```python
from build123d import *

# Parameters (mm, degrees)
EXTRUDE_THIN1_DEPTH = 317.5
FILLET1_R           = 1.27


with BuildPart() as part:
    # Sketch1 → Extrude-Thin1 (new body)
    with BuildSketch(Plane.XY):
        with BuildLine():
            Line((0, 31.75), (-11.90625, 31.75))
            ThreePointArc((-11.90625, 31.75), (-15.756503047, 28.743813262), (-13.773897059, 24.279411765))
            ThreePointArc((-13.773897059, 24.279411765), (-6.608099772, 17.466390137), (-3.96875, 7.9375))
            Line((-3.96875, 7.9375), (-4.7625, 7.9375))
            ThreePointArc((-4.7625, 7.9375), (-7.540625, 5.159375), (-4.7625, 2.38125))
            Line((-4.7625, 2.38125), (-3.96875, 2.38125))
            Line((-3.96875, 2.38125), (-3.96875, 0))
            Line((-3.96875, 0), (0, 0))
            Line((0, 0), (0, 1.27))
            Line((0, 1.27), (-2.69875, 1.27))
            Line((-2.69875, 1.27), (-2.69875, 3.65125))
            Line((-2.69875, 3.65125), (-4.7625, 3.65125))
            ThreePointArc((-4.7625, 3.65125), (-6.270625, 5.159375), (-4.7625, 6.6675))
            Line((-4.7625, 6.6675), (-2.7395407, 6.6675))
            ThreePointArc((-2.7395407, 6.6675), (-5.200957167, 17.569762939), (-13.17625, 25.4))
            ThreePointArc((-13.17625, 25.4), (-14.524422072, 28.435793018), (-11.90625, 30.48))
            Line((-11.90625, 30.48), (0, 30.48))
            Line((0, 30.48), (0, 31.75))
        make_face()
    extrude(amount=-EXTRUDE_THIN1_DEPTH)

    # Fillet1
    fillet1_edges = [part.edges().sort_by_distance(p)[0] for p in [
        (-3.96875, 0, -158.75),
        (-2.7395407, 6.6675, -158.75),
        (-2.69875, 3.65125, -158.75),
    ]]
    fillet(fillet1_edges, radius=FILLET1_R)


solid = part.part
```
Input: part model. Units: mm. Frame: model coordinates. A direction names the side the tool comes from. Give positions to 0.01 mm unless a question says otherwise; leave off trailing zeros. Write each loop counter-clockwise with the first axis right and the second up, starting at its lowest first coordinate (ties: lowest second). Pieces come first, ordered by that corner, then holes. Notation, with made-up numbers: (63.25, 1) - (77.25, 1) arc R32 ccw to (77.25, 33) - close; hole circle Ø7 at (60, -7.75). An arc over 180 degrees is marked (long way). Write item = value, one per line. Start each with the question number.
1) Pin query (flat end, axial travel): pin 1 (5 mm diameter, centred on y = 16, z = -145.5, fed in from -X); pin 2 (0.6 mm diameter, centred on y = 2, z = -81.5, fed in from +X); pin 3 (1 mm diameter, centred on x = -3, y = 5.5, fed in from -Z) (3 decimals); pin 4 (6 mm diameter, centred on y = 10, z = -56.5, fed in from -X). Return the tip coordinate at first contact, or that it passes through.
2) Cut plane B-B (y = 12). Return loops of the section in (x, z).
3) Cut plane A-A (z = -274). Return loops of the section in (x, y), and give its area (3 significant figures).
4) Material intervals for L1, parallel to Y at x = -5.5, z = -208.5; L2, parallel to Y at x = -1, z = -225.5; L3, parallel to Y at x = -5.75, z = -82, sorted ascending. Write a range as [from, to].
5) Draft query along Y for faces 4 (the face through (-15.738, 28.815, -156.528)), 5 (the face through (-7.54, 5.22, -156.53)), 6 (the face through (-7, 19, 0)). Return one class per face: pulls with the +Y half, pulls with the -Y half, needs draft (parallel to the pull), parting line crosses it, or undercut.
6) Reachability of faces 1 (the face through (-6.681, 17.586, -156.528)), 2 (the face through (-7, 19, -317.5)), 3 (the face through (-5.44, 17.99, -156.53)) from +Z, -Z, +X, -X, +Y, -Y: full face, straight path, thin tool, end or side. Return the list, or none.
Answers follow:
q1.pin_1 = -7.28
q1.pin_2 = -2.7
q1.pin_3 = through
q1.pin_4 = -6.84
q2.outline = (-4.42, -317.5) - (-3.12, -317.5) - (-3.12, 0) - (-4.42, 0) - close
q3.outline = (-13.77, 24.28) arc R18.52 cw to (-3.97, 7.94) - (-4.76, 7.94) arc R2.78 ccw to (-4.76, 2.38) - (-3.97, 2.38) - (-3.97, 1.27) arc R1.27 ccw to (-2.7, 0) - (0, 0) - (0, 1.27) - (-2.7, 1.27) - (-2.7, 2.38) arc R1.27 ccw to (-3.97, 3.65) - (-4.76, 3.65) arc R1.51 cw to (-4.76, 6.67) - (-3.97, 6.67) arc R1.27 ccw to (-2.7, 7.94) arc R19.79 ccw to (-13.18, 25.4) arc R2.7 cw to (-11.91, 30.48) - (0, 30.48) - (0, 31.75) - (-11.91, 31.75) arc R3.97 ccw to start
q3.area = 71.8 mm^2
q4.L1 = [2.48, 3.84], [6.47, 7.84], [15.31, 18.09], [30.48, 31.75]
q4.L2 = [0, 1.27], [30.48, 31.75]
q4.L3 = [2.56, 4.02], [6.3, 7.76], [15.86, 18.5], [30.48, 31.75]
q5.face_4 = parting line crosses it
q5.face_5 = undercut
q5.face_6 = needs draft
q6.face_1 = +Z, -Z, -X
q6.face_2 = -Z, +X, -X, +Y, -Y
q6.face_3 = +Z, -Z, +X
